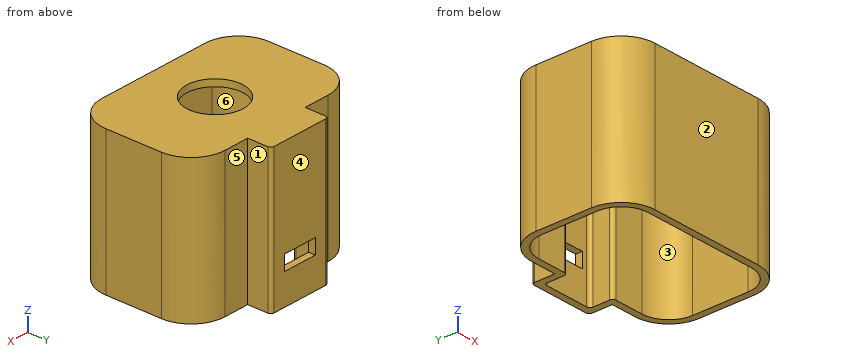
```python
from build123d import *

# Parameters (mm, degrees)
F1_DEPTH = 63.5
F2_W     = 16.383
F2_H     = 6.985
F3_DEPTH = 3.175
F4_R     = 1.5875
F6_DEPTH = 3.175
F7_R     = 13.2842
F8_DEPTH = 3.175


with BuildPart() as f1:
    # F0 (on Top) → F1 (new body)
    with BuildSketch(Plane.XY):
        with BuildLine():
            Line((-15.24, 40.005), (-15.24, 28.956))
            Line((-15.24, 28.956), (-27.305, 28.956))
            ThreePointArc((-27.305, 28.956), (-38.53032, 24.30632), (-43.18, 13.081))
            Line((-43.18, 13.081), (-43.18, -13.081))
            ThreePointArc((-43.18, -13.081), (-38.53032, -24.30632), (-27.305, -28.956))
            Line((-27.305, -28.956), (27.305, -28.956))
            ThreePointArc((27.305, -28.956), (38.53032, -24.30632), (43.18, -13.081))
            Line((43.18, -13.081), (43.18, 13.081))
            ThreePointArc((43.18, 13.081), (38.53032, 24.30632), (27.305, 28.956))
            Line((27.305, 28.956), (15.24, 28.956))
            Line((15.24, 28.956), (15.24, 40.005))
            Line((15.24, 40.005), (-15.24, 40.005))
        make_face()
        with BuildLine():
            Line((12.065, 25.781), (27.305, 25.781))
            ThreePointArc((27.305, 25.781), (36.285256, 22.061256), (40.005, 13.081))
            Line((40.005, 13.081), (40.005, -13.081))
            ThreePointArc((40.005, -13.081), (36.285256, -22.061256), (27.305, -25.781))
            Line((27.305, -25.781), (-27.305, -25.781))
            ThreePointArc((-27.305, -25.781), (-36.285256, -22.061256), (-40.005, -13.081))
            Line((-40.005, -13.081), (-40.005, 13.081))
            ThreePointArc((-40.005, 13.081), (-36.285256, 22.061256), (-27.305, 25.781))
            Line((-27.305, 25.781), (-12.065, 25.781))
            Line((-12.065, 25.781), (-12.065, 36.83))
            Line((-12.065, 36.83), (12.065, 36.83))
            Line((12.065, 36.83), (12.065, 25.781))
        make_face(mode=Mode.SUBTRACT)
    extrude(amount=F1_DEPTH)

    # F2 (on face) → F3 (cut, through all)
    with BuildSketch(Plane(origin=(0, 40.005, 0), x_dir=(-1, 0, 0), z_dir=(0, 1, 0))):
        with Locations((0, 17.8435)):
            Rectangle(F2_W, F2_H)
    extrude(amount=-F3_DEPTH, mode=Mode.SUBTRACT)

    # F4
    f4_edges = [f1.edges().sort_by_distance(p)[0] for p in [
        (-12.065, 25.781, 31.75),
        (-12.065, 36.83, 31.75),
        (12.065, 25.781, 31.75),
        (12.065, 36.83, 31.75),
        (15.24, 40.005, 31.75),
        (-15.24, 40.005, 31.75),
    ]]
    fillet(f4_edges, radius=F4_R)

    # F5 (on face) → F6 (join)
    with BuildSketch(Plane.XY.offset(63.5)):
        with BuildLine():
            Line((13.6525, 40.005), (-13.6525, 40.005))
            ThreePointArc((-13.6525, 40.005), (-14.775032, 39.540032), (-15.24, 38.4175))
            Line((-15.24, 38.4175), (-15.24, 28.956))
            Line((-15.24, 28.956), (-27.305, 28.956))
            ThreePointArc((-27.305, 28.956), (-38.53032, 24.30632), (-43.18, 13.081))
            Line((-43.18, 13.081), (-43.18, -13.081))
            ThreePointArc((-43.18, -13.081), (-38.53032, -24.30632), (-27.305, -28.956))
            Line((-27.305, -28.956), (27.305, -28.956))
            ThreePointArc((27.305, -28.956), (38.53032, -24.30632), (43.18, -13.081))
            Line((43.18, -13.081), (43.18, 13.081))
            ThreePointArc((43.18, 13.081), (38.53032, 24.30632), (27.305, 28.956))
            Line((27.305, 28.956), (15.24, 28.956))
            Line((15.24, 28.956), (15.24, 38.4175))
            ThreePointArc((15.24, 38.4175), (14.775032, 39.540032), (13.6525, 40.005))
        make_face()
    extrude(amount=F6_DEPTH)

    # F7 (on face) → F8 (cut, through all)
    with BuildSketch(Plane.XY.offset(66.675)):
        Circle(F7_R)
    extrude(amount=-F8_DEPTH, mode=Mode.SUBTRACT)


with BuildPart() as f9_1:
    # F9: copy of F1
    add(f1.part)


solid = f1.part
```
Design review of the part built by this model. Coordinates are the model's own, in mm. Face numbers are marked on the shaded views. A direction names the side the tool comes from. Coordinates: 2 decimals unless noted, no trailing zeros. Order: outer loops, then holes, each group sorted by start corner. A loop starts at its lowest first (then second) coordinate and runs counter-clockwise, first axis right, second up. Notation, with made-up numbers: (20.25, 60) -> (41.25, 60) arc R8 ccw to (41.25, 71) -> close; hole circle Ø3 at (47.25, -16). An arc over 180 degrees is marked (long way). One line per item, written item: value. Start each with the question number.
Q1. Take a section at A-A, the plane x = 0. State the section outline as (y, z) points (3 decimals), then the cut area to 3 significant figures.
Q2. Take a section at C-C, the plane y = -3.5. State the section outline as (x, z) points (3 decimals), then the cut area to 3 significant figures.
Q3. For probe 1 along X at (y, z) = (30.5, 9.5) (3 decimals); probe 2 along X at (y, z) = (-8, 53) (3 decimals); probe 3 along Y at (x, z) = (0, 65.4) (3 decimals), list the stretches that pass through material, from the lowest coordinate up.
Q4. Mouldability with a two-part tool opening along X and no side actions: class the marked faces 1, 2 and 3 as pulls with the +X half, pulls with the -X half, needs draft (parallel to the pull), parting line crosses it, or undercut.
Q5. Take a section at D-D, the plane y = 24. State the section outline as (x, z) points (1 decimal).
Q6. Tool access review of the marked faces 4, 5 and 6: name each direction out of +Z, -Z, +X, -X, +Y, -Y from which nothing blocks a thin tool from reaching the whole face with its end or side.
Q7. Insertion check: pin 1 Ø3.5 at (x, z) = (19.5, 43.5) entering from +Y; pin 2 Ø2.5 at (y, z) = (32.5, 30.5) entering from +X; pin 3 Ø1.5 at (x, y) = (7.5, 15) entering from -Z. Each pin has a flat end and moves straight along its axis. Give the tip position at first contact, or say it passes through.
Values follow:
1. outline: (-28.956, 0) -> (-25.781, 0) -> (-25.781, 63.5) -> (-13.284, 63.5) -> (-13.284, 66.675) -> (-28.956, 66.675) -> close; (13.284, 63.5) -> (36.83, 63.5) -> (36.83, 21.336) -> (40.005, 21.336) -> (40.005, 66.675) -> (13.284, 66.675) -> close; (36.83, 0) -> (40.005, 0) -> (40.005, 14.351) -> (36.83, 14.351) -> close
1. area: 516 mm2
2. outline: (-43.18, 0) -> (-40.005, 0) -> (-40.005, 63.5) -> (-12.815, 63.5) -> (-12.815, 66.675) -> (-43.18, 66.675) -> close; (12.815, 63.5) -> (40.005, 63.5) -> (40.005, 0) -> (43.18, 0) -> (43.18, 66.675) -> (12.815, 66.675) -> close
2. area: 596 mm2
3. probe 1: x = -15.24 to -12.065, 12.065 to 15.24
3. probe 2: x = -43.18 to -40.005, 40.005 to 43.18
3. probe 3: y = -28.956 to -13.284, 13.284 to 40.005
4. face 1: pulls with the +X half
4. face 2: needs draft
4. face 3: undercut
5. outline: (-38.8, 0) -> (-33.8, 0) -> (-33.8, 63.5) -> (33.8, 63.5) -> (33.8, 0) -> (38.8, 0) -> (38.8, 66.7) -> (-38.8, 66.7) -> close
6. face 4: +Z, -Z, +X, -X, +Y
6. face 5: +Z, -Z, +X, +Y
6. face 6: -Z
7. pin 1: stops at y = 28.96
7. pin 2: stops at x = 15.24
7. pin 3: stops at z = 63.5
